Design review of the part built by this model. Coordinates are the model's own, in mm. Round coordinates to 2 decimals unless told otherwise and drop trailing zeros. Write each loop counter-clockwise with the first axis right and the second up, starting at its lowest first coordinate (ties: lowest second). Pieces come first, ordered by that corner, then holes. Notation, with made-up numbers: (61.25, 36.5) - (70.25, 36.5) arc R22 ccw to (70.25, 66.5) - close; hole circle Ø11 at (89.25, 28.25). An arc over 180 degrees is marked (long way). Use one line per item in the form item = value.
Autodesk Inventor part; units mm, degrees
ref_plane "YZ Plane" through (0, 0, 0) normal (1, 0, 0) x (0, 1, 0)
ref_plane "XZ Plane" through (0, 0, 0) normal (0, 1, 0) x (-1, 0, 0)
ref_plane "XY Plane" through (0, 0, 0) normal (0, 0, 1) x (1, 0, 0)
sketch "Sketch1" plane through (0, 0, 0) normal (0, 0, 1) x (1, 0, 0)
  line L0 (-17.5, 15) -> (17.5, 15)
  line L1 (17.5, 15) -> (17.5, -15)
  line L2 (17.5, -15) -> (-17.5, -15)
  line L3 (-17.5, -15) -> (-17.5, 15)
  point P0 (0, 0)
  point P1 (0, 15)
  point P2 (-17.5, 0)
  dimension "d0" = 35
  dimension "d1" = 30
extrude "Extrusion1" add sketch "Sketch1" along normal blind 8
sketch "Sketch6" plane through (0, 0, 8) normal (0, 0, 1) x (1, 0, 0)
  circle A0 centre (5.7312, -11.8725) radius 1.7875
  circle A1 centre (-13.4438, -11.8725) radius 1.7875
  point P0 (0, 0)
hole "Hole1" at (5.7312, -11.8725, 8) at (-13.4438, -11.8725, 8) direction (0, 0, -1) diameter 2.459 end through all
properties part number "0005-10-028 suport senzor y"
Q1. We need section A-A on y = -12. Write out the cut boundary in (x, z).
Calculated:
outline = (-17.5, 0) - (-14.67, 0) - (-14.67, 8) - (-17.5, 8) - close; (-12.22, 0) - (4.51, 0) - (4.51, 8) - (-12.22, 8) - close; (6.95, 0) - (17.5, 0) - (17.5, 8) - (6.95, 8) - close
Q2. Draft analysis for pull direction X (two halves, no side actions). For faces 1 (the flat face through (17.5, 0, 4)), 2 (the cylindrical face through (6.82, -12.44, 3.94)), 3 (the flat face through (0, 0, 0)), state which applies: released by +X, released by -X, zero draft, split by the parting line, or undercut.
Calculated:
face_1 = released by +X
face_2 = undercut
face_3 = zero draft
Q3. To check wall thickness, follow line 1 along X through (y, z) = (-11.75, 2.5); line 2 along X through (y, z) = (-10.75, 6); line 3 along Y through (x, z) = (-14.5, 6). State the ranges of each line that lie inside material, in increasing order. Write a range as from..to.
Calculated:
line_1 = -17.5..-14.67, -12.22..4.51, 6.95..17.5
line_2 = -17.5..-13.95, -12.94..5.23, 6.23..17.5
line_3 = -15..-12.5, -11.24..15
